from build123d import *

# Parameters (mm, degrees)
F1_DEPTH      = 1.75
F1_DEPTH_BACK = 1.75
F3_DEPTH      = 25


with BuildPart() as f1:
    # F0 (on Front) → F1 (new body, two sides)
    with BuildSketch(Plane.XZ) as f1_sk:
        with BuildLine():
            Line((0.595, 0.15), (-2.655, 0.15))
            Line((-2.655, 0.15), (-2.655, 0))
            Line((-2.655, 0), (0.745, 0))
            ThreePointArc((0.745, 0), (0.815711, 0.029289), (0.845, 0.1))
            Line((0.845, 0.1), (0.845, 5.05))
            ThreePointArc((0.845, 5.05), (0.903579, 5.191421), (1.045, 5.25))
            Line((1.045, 5.25), (1.612098, 5.25))
            ThreePointArc((1.612098, 5.25), (1.732534, 5.209672), (1.804401, 5.104952))
            Line((1.804401, 5.104952), (2.352996, 3.185167))
            ThreePointArc((2.352996, 3.185167), (2.352908, 3.129908), (2.323486, 3.083132))
            Line((2.323486, 3.083132), (2.129785, 2.91))
            Line((2.129785, 2.91), (2.279785, 2.91))
            Line((2.279785, 2.91), (2.478268, 3.087407))
            ThreePointArc((2.478268, 3.087407), (2.50769, 3.134182), (2.507779, 3.189441))
            Line((2.507779, 3.189441), (1.917541, 5.254952))
            ThreePointArc((1.917541, 5.254952), (1.845674, 5.359672), (1.725239, 5.4))
            Line((1.725239, 5.4), (0.895, 5.4))
            ThreePointArc((0.895, 5.4), (0.753579, 5.341421), (0.695, 5.2))
            Line((0.695, 5.2), (0.695, 2.91))
            Line((0.695, 2.91), (0.695, 0.25))
            ThreePointArc((0.695, 0.25), (0.665711, 0.179289), (0.595, 0.15))
        make_face()
    extrude(amount=F1_DEPTH)
    extrude(f1_sk.sketch, amount=-F1_DEPTH_BACK)

    # F2 (on face) → F3 (cut)
    with BuildSketch(Plane.YZ.offset(0.845)):
        with BuildLine():
            Line((-0.58, 4.004952), (-0.58, 2.610195))
            Line((-0.58, 2.610195), (0.58, 2.610195))
            Line((0.58, 2.610195), (0.58, 4.004952))
            ThreePointArc((0.58, 4.004952), (0.433553, 4.358506), (0.08, 4.504952))
            Line((0.08, 4.504952), (-0.08, 4.504952))
            ThreePointArc((-0.08, 4.504952), (-0.433553, 4.358506), (-0.58, 4.004952))
        make_face()
    extrude(amount=F3_DEPTH, mode=Mode.SUBTRACT)


solid = f1.part
CAD build for the part. Positions are in the model's coordinates, mm. A direction names the side the tool comes from. Round coordinates to 2 decimals unless told otherwise and drop trailing zeros. Loops run counter-clockwise (first coordinate to the right, second up) from the corner with the lowest first, then second, coordinate; pieces in that order, holes last. Notation, with made-up numbers: M -16,21 L 41,21 A20 ccw 41,59 Z; hole C 39.25,89 d2. An arc over 180 degrees is marked long. One line per question, with ' | ' between items. Start each with the question number.
Item 1: Cut at A-A, the plane z = 4.2. Write the cut outline in (x, y) (3 decimals).
Item 2: Which spindle directions (+Z, -Z, +X, -X, +Y, -Y) get a long thin tool onto all of the face, cutting with end or side? Do faces 1 (the flat face through (1.95, -0.41, 4.59)), 2 (the flat face through (0.845, 0, 3)), 3 (the flat face through (0.695, 0, 3)). Say none if no direction does.
Item 3: Pin check, flat tips, straight feed: pin 1 Ø1.8 at (y, z) = (-0.5, 3.5) entering from -X (3 decimals); pin 2 Ø1 at (x, y) = (-1.5, 0.5) entering from +Z; pin 3 Ø1.5 at (x, z) = (-0.5, 3.5) entering from -Y. Stop position of each tip, or through.
Item 4: Cut at C-C, the plane x = -1.5. Write the cut outline in (y, z).
Item 5: Cut at D-D, the plane z = 0.75. Write the cut outline in (x, y) (3 decimals), plus the area to 3 significant figures.
Item 6: Wall check: line 1 (X direction, y = -0.7, z = 0.95) (3 decimals); line 2 (Z direction, x = 1.5, y = 0.6); line 3 (X direction, y = -0.7, z = 3.35) (3 decimals). Give the ranges that are in metal, low to high.
Item 7: Cut at B-B, the plane y = -0.8. Write the cut outline in (x, z) (3 decimals).
Responses:
1) outline: M 0.695,-1.75 L 0.845,-1.75 L 0.845,1.75 L 0.695,1.75 Z; M 2.063,-1.75 L 2.219,-1.75 L 2.219,-0.54 L 2.063,-0.54 Z; M 2.063,0.54 L 2.219,0.54 L 2.219,1.75 L 2.063,1.75 Z
2) face 1: +Y, -Y | face 2: -Z, +Y, -Y | face 3: +Z, -X, +Y, -Y
3) pin 1: stops at x = 0.695 | pin 2: stops at z = 0.15 | pin 3: passes through
4) outline: M -1.75,0 L 1.75,0 L 1.75,0.15 L -1.75,0.15 Z
5) outline: M 0.695,-1.75 L 0.845,-1.75 L 0.845,1.75 L 0.695,1.75 Z | area: 0.525 mm²
6) line 1: x = 0.695 to 0.845 | line 2: z = 5.25 to 5.4 | line 3: x = 0.695 to 0.845, 2.306 to 2.462
7) outline: M -2.655,0 L 0.745,0 A0.1 ccw 0.845,0.1 L 0.845,5.05 A0.2 cw 1.045,5.25 L 1.612,5.25 A0.2 cw 1.804,5.105 L 2.353,3.185 A0.1 cw 2.323,3.083 L 2.13,2.91 L 2.28,2.91 L 2.478,3.087 A0.1 ccw 2.508,3.189 L 1.918,5.255 A0.2 ccw 1.725,5.4 L 0.895,5.4 A0.2 ccw 0.695,5.2 L 0.695,0.25 A0.1 cw 0.595,0.15 L -2.655,0.15 Z
